from build123d import *

# Parameters (mm, degrees)
SKETCH1_W           = 10
SKETCH1_H           = 18
BOSS_EXTRUDE1_DEPTH = 1.6
BOSS_EXTRUDE2_DEPTH = 7


with BuildPart() as part:
    # Sketch1 → Boss-Extrude1 (new body)
    with BuildSketch(Plane(origin=(0, 0, 0), x_dir=(1, 0, 0), z_dir=(0, 1, 0))):
        with Locations((5, 9)):
            Rectangle(SKETCH1_W, SKETCH1_H)
    extrude(amount=BOSS_EXTRUDE1_DEPTH)

    # Sketch3 → Boss-Extrude2 (add)
    with BuildSketch(Plane.XY.offset(1)):
        with BuildLine():
            Line((1.87, 4.74), (8.13, 4.74))
            ThreePointArc((8.13, 4.74), (9.028025612, 4.368025612), (9.4, 3.47))
            Line((9.4, 3.47), (9.4, 2.87))
            ThreePointArc((9.4, 2.87), (9.028025612, 1.971974388), (8.13, 1.6))
            Line((8.13, 1.6), (1.87, 1.6))
            ThreePointArc((1.87, 1.6), (0.971974388, 1.971974388), (0.6, 2.87))
            Line((0.6, 2.87), (0.6, 3.47))
            ThreePointArc((0.6, 3.47), (0.971974388, 4.368025612), (1.87, 4.74))
        make_face()
    extrude(amount=-BOSS_EXTRUDE2_DEPTH)


solid = part.part
Here's how the part is built. I have some questions about the finished solid (model axes, mm). A direction names the side the tool comes from. Round coordinates to 2 decimals unless told otherwise and drop trailing zeros. Order: outer loops, then holes, each group sorted by start corner. A loop starts at its lowest first (then second) coordinate and runs counter-clockwise, first axis right, second up. Notation, with made-up numbers: (23, 19.5) -> (72, 19.5) arc R25 cw to (72, 45.5) -> close; hole circle Ø1 at (-15.75, -4.75). An arc over 180 degrees is marked (long way). Use CSV: the item, a comma, the result in double quotes.
1. I want a section at A-A on z = -0.25. List the corners of the cut face in (x, y) for me.
Recorded:
outline,"(0, 0) -> (10, 0) -> (10, 1.6) -> (8.13, 1.6) arc R1.27 ccw to (9.4, 2.87) -> (9.4, 3.47) arc R1.27 ccw to (8.13, 4.74) -> (1.87, 4.74) arc R1.27 ccw to (0.6, 3.47) -> (0.6, 2.87) arc R1.27 ccw to (1.87, 1.6) -> (0, 1.6) -> close"
2. Which directions (+Z, -Z, +X, -X, +Y, -Y) give clear straight access to the entire face, cutting with the end or side of a thin tool? Please do faces 1 (the face through (5, 1.6, 0.5)), 2 (the face through (0, 1, -9)).
Recorded:
face 1,"+Z, +X, -X, -Y"
face 2,"+Z, -Z, -X, +Y, -Y"
3. I want a section at C-C on x = 3.25. List the corners of the cut face in (y, z) for me, and give its area (3 significant figures).
Recorded:
outline,"(0, -18) -> (1.6, -18) -> (1.6, -6) -> (4.74, -6) -> (4.74, 1) -> (1.6, 1) -> (1.6, 0) -> (0, 0) -> close"
area,"50.8 mm2"
4. I want a section at B-B on x = 8.5. List the corners of the cut face in (y, z) for me, and give its area (3 significant figures).
Recorded:
outline,"(0, -18) -> (1.6, -18) -> (1.6, 0) -> (0, 0) -> close; (1.66, -6) -> (4.68, -6) -> (4.68, 1) -> (1.66, 1) -> close"
area,"50.0 mm2"
5. I need wall thicknesses on line 1 along Z through (x, y) = (4.75, 4.1); line 2 along Y through (x, z) = (2.25, -7.75); line 3 along Z through (x, y) = (6.25, 0.4). Which ranges of each line are inside material? Lowest first, please.
Recorded:
line 1,"z = -6 to 1"
line 2,"y = 0 to 1.6"
line 3,"z = -18 to 0"
6. I'm going to push flat-ended pins straight in: P1, Ø0.5, axis at x = 6.5, y = 0.5, coming from the +Z side; P2, Ø1.5, axis at y = 3.5, z = -12.5, coming from the +X side; P3, Ø0.8, axis at x = 4.5, z = 0.5, coming from the -Y side; P4, Ø3, axis at x = 7, z = -12, coming from the -Y side. Where does each tip first touch, or does it pass through?
Recorded:
P1,"stops at z = 0"
P2,"passes through"
P3,"stops at y = 1.6"
P4,"stops at y = 0"
7. Thinking about a two-plate mould opening in Y: for faces 3 (the face through (5, 3, -6)), 4 (the face through (5, 0, -9)), 5 (the face through (0.982, 1.962, -2.451)), which applies, pulls with the +Y half, pulls with the -Y half, needs draft (parallel to the pull), parting line crosses it, or undercut?
Recorded:
face 3,"needs draft"
face 4,"pulls with the -Y half"
face 5,"undercut"
8. I want a section at D-D on y = 0.3. List the corners of the cut face in (x, z) for me, and give its area (3 significant figures).
Recorded:
outline,"(0, -18) -> (10, -18) -> (10, 0) -> (0, 0) -> close"
area,"180 mm2"
